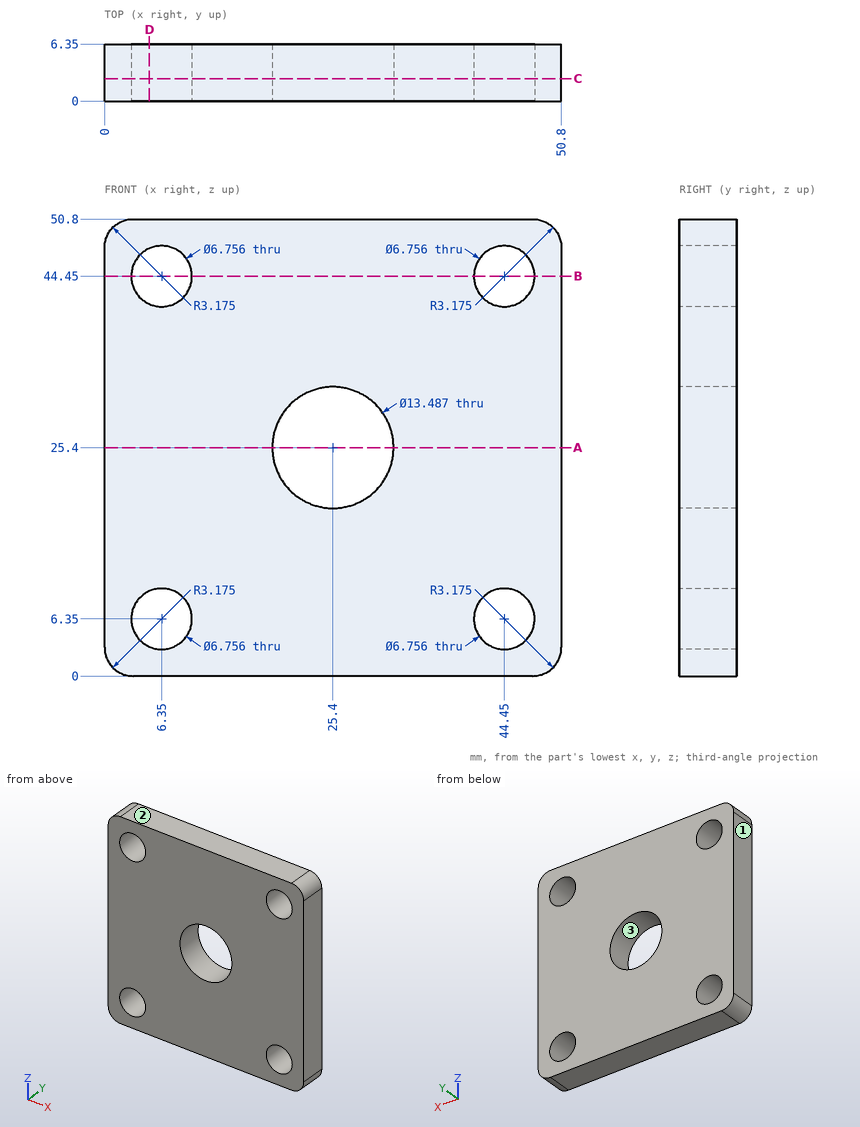
Part print with two shaded views. Sizes in mm from the minimum x, y, z corner. Round coordinates to 2 decimals unless told otherwise and drop trailing zeros. Order: outer loops, then holes, each group sorted by start corner. A loop starts at its lowest first (then second) coordinate and runs counter-clockwise, first axis right, second up. Notation, with made-up numbers: (32.25, 58) - (45.25, 58) arc R25 cw to (45.25, 95) - close; hole circle Ø7 at (68, 4.25). An arc over 180 degrees is marked (long way). Return JSON: item names as keys, results as strings.
(1) Wall check: probe 1 along X at (y, z) = (4, 6.35); probe 2 along X at (y, z) = (4, 42) (1 decimal). Give the ranges that are in metal, low to high. Write a range as from..to.
Answer key:
{"probe 1": "x = 0..2.97, 9.73..41.07, 47.83..50.8", "probe 2": "x = 0..4, 8.7..42.1, 46.8..50.8"}
(2) Cut at C-C (y = 2.5). State how many separate pieces and enclosed holes the cut face has, then the cut area to 3 significant figures.
Answer key:
{"separate pieces": "1", "enclosed holes": "5", "area": "2,290 mm^2"}
(3) Cut at D-D (x = 5). Give the cut face in (y, z), then the cut area to 3 significant figures.
Answer key:
{"outline": "(0, 0) - (6.35, 0) - (6.35, 3.25) - (0, 3.25) - close; (0, 9.45) - (6.35, 9.45) - (6.35, 41.35) - (0, 41.35) - close; (0, 47.55) - (6.35, 47.55) - (6.35, 50.8) - (0, 50.8) - close", "area": "244 mm^2"}
(4) Pull direction X, two halves, no side cores. Call the marked faces 1, 2 and 3: +X half, -X half, draft (parallel to the pull), parting line (faces both ways), or undercut.
Answer key:
{"face 1": "-X half", "face 2": "draft", "face 3": "undercut"}
(5) Cut at A-A (z = 25.4). Give the cut face in (x, y).
Answer key:
{"outline": "(0, 0) - (18.66, 0) - (18.66, 6.35) - (0, 6.35) - close; (32.14, 0) - (50.8, 0) - (50.8, 6.35) - (32.14, 6.35) - close"}
(6) Cut at B-B (z = 44.45). Give the cut face in (x, y).
Answer key:
{"outline": "(0, 0) - (2.97, 0) - (2.97, 6.35) - (0, 6.35) - close; (9.73, 0) - (41.07, 0) - (41.07, 6.35) - (9.73, 6.35) - close; (47.83, 0) - (50.8, 0) - (50.8, 6.35) - (47.83, 6.35) - close"}
